from build123d import *

# Parameters (mm, degrees)
SKETCH1_R          = 5.25
SKETCH1_R_2        = 2.25
BASE_FLANGE1_DEPTH = 0.75
CHAMFER1_SIZE      = 0.025


# Sheet-metal steps are written as plain solids
with BuildPart() as part:
    # Sketch1 → Base-Flange1 (new body)
    with BuildSketch(Plane.XY):
        Circle(SKETCH1_R)
        Circle(SKETCH1_R_2, mode=Mode.SUBTRACT)
    extrude(amount=-BASE_FLANGE1_DEPTH)

    # Chamfer1
    chamfer1_edges = [part.edges().sort_by_distance(p)[0] for p in [
        (-5.25, 0, 0),
        (-5.25, 0, -0.75),
        (-2.25, 0, -0.75),
        (-2.25, 0, 0),
    ]]
    chamfer(chamfer1_edges, length=CHAMFER1_SIZE)


solid = part.part
Verification items for the finished model (mm, model axes). Give positions to 0.01 mm unless a question says otherwise; leave off trailing zeros. Order: outer loops, then holes, each group sorted by start corner. A loop starts at its lowest first (then second) coordinate and runs counter-clockwise, first axis right, second up. Notation, with made-up numbers: M 43,23.5 L 49,23.5 A29 cw 49,48.5 Z; hole C -8,1 d10. An arc over 180 degrees is marked long. Use one line per item in the form item = value. Start each with the question number.
Q1. Mould release check, pull along Y, two halves, no side actions. Record for faces 1 (the cylindrical face through (5, 1.6, -0.4)), 2 (the flat face through (2.2, -1.1, -0.75)), 3 (the cylindrical face through (-0.29, 2.23, -0.37)): +Y half, -Y half, draft (parallel to the pull), parting line (faces both ways), or undercut.
Q2. Section check C-C (z = -0.2). Enter the section's corners in (x, y).
Q3. Scan lines: line 1 along Y through (x, z) = (0, -0.4); line 2 along Y through (x, z) = (-1, -0.4); line 3 along X through (y, z) = (2, -0.35). Record each from-to range of solid material in increasing order. Write a range as [from, to].
Q4. Section check A-A (x = 0). Enter the section's corners in (y, z) (3 decimals).
Evaluation:
q1.face_1 = parting line
q1.face_2 = draft
q1.face_3 = undercut
q2.outline = C 0,0 d10.5; hole C 0,0 d4.5
q3.line_1 = [-5.25, -2.25], [2.25, 5.25]
q3.line_2 = [-5.15, -2.02], [2.02, 5.15]
q3.line_3 = [-4.85, -1.03], [1.03, 4.85]
q4.outline = M -5.25,-0.725 L -5.225,-0.75 L -2.275,-0.75 L -2.25,-0.725 L -2.25,-0.025 L -2.275,0 L -5.225,0 L -5.25,-0.025 Z; M 2.25,-0.725 L 2.275,-0.75 L 5.225,-0.75 L 5.25,-0.725 L 5.25,-0.025 L 5.225,0 L 2.275,0 L 2.25,-0.025 Z
